```python
from build123d import *

# Parameters (mm, degrees)
SKETCH_1_R          = 7
EXTRUDE_1_DEPTH     = 3
SKETCH_2_R          = 6
EXTRUDE_2_DEPTH     = 8
SKETCH_3_R          = 7
EXTRUDE_3_DEPTH     = 3
CHAMFER_1_SIZE      = 2.144506921
CHAMFER_1_SIZE_2    = 1
CHAMFER_2_SIZE      = 2.144506921
CHAMFER_2_SIZE_2    = 1
SKETCH_4_R          = 5.9
EXTRUDE_4_DEPTH     = 2.2
EXTRUDE_START       = 2.2
SKETCH_5_R          = 5.9
EXTRUDE_5_DEPTH     = 2.2
SKETCH_6_W          = 6.5
SKETCH_6_H          = 6.5
CUT_EXTRUDE_1_DEPTH = 4
SKETCH_7_W          = 6.5
SKETCH_7_H          = 6.5
CUT_EXTRUDE_2_DEPTH = 4
SKETCH_8_R          = 1.2
CUT_EXTRUDE_3_DEPTH = 18.474552927


with BuildPart() as part:
    # Эскиз1 → Бобышка-Вытянуть1 (new body)
    with BuildSketch(Plane(origin=(0, 0, 0), x_dir=(1, 0, 0), z_dir=(0, 1, 0))):
        with Locations(Location((0, 0, 0), (0, 0, 270))):
            Circle(SKETCH_1_R)
    extrude(amount=EXTRUDE_1_DEPTH)

    # Эскиз2 → Бобышка-Вытянуть2 (add)
    with BuildSketch(Plane(origin=(0, 3, 0), x_dir=(1, 0, 0), z_dir=(0, 1, 0))):
        with Locations(Location((0, 0, 0), (0, 0, 270))):
            Circle(SKETCH_2_R)
    extrude(amount=EXTRUDE_2_DEPTH)

    # Эскиз3 → Бобышка-Вытянуть3 (add)
    with BuildSketch(Plane(origin=(0, 11, 0), x_dir=(1, 0, 0), z_dir=(0, 1, 0))):
        with Locations(Location((0, 0, 0), (0, 0, 270))):
            Circle(SKETCH_3_R)
    extrude(amount=EXTRUDE_3_DEPTH)

    # Фаска1
    # the kernel refuses this chamfer: 2.144506921, 1 mm, written as the material it adds along each edge
    with BuildSketch(Plane(origin=(0, 3, 0), x_dir=(0, 0, 1), z_dir=(-1, 0, 0))) as chamfer_1_piece_1_section:
        Polygon((6, CHAMFER_1_SIZE), (6 + CHAMFER_1_SIZE_2, 0), (6, 0), align=None)
    chamfer_1_piece_1 = revolve(axis=Axis((0, 3, 0), (0, 1, 0)), mode=Mode.PRIVATE)
    chamfer_1_piece_1 = chamfer_1_piece_1 & Plane(origin=(0, 4.095664656, 0), x_dir=(0, 0, 1), z_dir=(0, -1, 0)) * Cylinder(7, 28, mode=Mode.PRIVATE)
    add(chamfer_1_piece_1)

    # Фаска2
    # the kernel refuses this chamfer: 2.144506921, 1 mm, written as the material it adds along each edge
    with BuildSketch(Plane(origin=(0, 11, 0), x_dir=(0, 0, 1), z_dir=(-1, 0, 0))) as chamfer_2_piece_1_section:
        Polygon((6, -CHAMFER_2_SIZE), (6 + CHAMFER_2_SIZE_2, 0), (6, 0), align=None)
    chamfer_2_piece_1 = revolve(axis=Axis((0, 11, 0), (0, 1, 0)), mode=Mode.PRIVATE)
    chamfer_2_piece_1 = chamfer_2_piece_1 & Plane(origin=(0, 9.904335344, 0), x_dir=(0, 0, 1), z_dir=(0, -1, 0)) * Cylinder(7, 28, mode=Mode.PRIVATE)
    add(chamfer_2_piece_1)

    # Эскиз4 → Бобышка-Вытянуть4 (add)
    with BuildSketch(Plane(origin=(0, 14, 0), x_dir=(1, 0, 0), z_dir=(0, 1, 0))):
        with Locations(Location((0, 0, 0), (0, 0, 270))):
            Circle(SKETCH_4_R)
    extrude(amount=EXTRUDE_4_DEPTH)

    # Эскиз5 → Бобышка-Вытянуть5 (add)
    with BuildSketch(Plane.XZ.offset(EXTRUDE_START)):
        with Locations(Location((0, 0, 0), (0, 0, 90))):
            Circle(SKETCH_5_R)
    extrude(amount=-EXTRUDE_5_DEPTH)

    # Эскиз6 → Вырез-Вытянуть1 (cut)
    with BuildSketch(Plane(origin=(0, 16.2, 0), x_dir=(1, 0, 0), z_dir=(0, 1, 0))):
        Rectangle(SKETCH_6_W, SKETCH_6_H)
    extrude(amount=-CUT_EXTRUDE_1_DEPTH, mode=Mode.SUBTRACT)

    # Эскиз7 → Вырез-Вытянуть2 (cut)
    with BuildSketch(Plane.XZ.offset(2.2)):
        Rectangle(SKETCH_7_W, SKETCH_7_H)
    extrude(amount=-CUT_EXTRUDE_2_DEPTH, mode=Mode.SUBTRACT)

    # Эскиз8 → Вырез-Вытянуть3 (cut, through all)
    with BuildSketch(Plane.XZ.offset(-1.8)):
        with Locations(Location((0, 0, 0), (0, 0, 270))):
            Circle(SKETCH_8_R)
    extrude(amount=-CUT_EXTRUDE_3_DEPTH, mode=Mode.SUBTRACT)


solid = part.part
```
Verification items for the finished model (mm, model axes). A direction names the side the tool comes from. Coordinates: 2 decimals unless noted, no trailing zeros. Write each loop counter-clockwise with the first axis right and the second up, starting at its lowest first coordinate (ties: lowest second). Pieces come first, ordered by that corner, then holes. Notation, with made-up numbers: M 17,-11 L 67,-11 A23 cw 67,2 Z; hole C 76.25,30 d10. An arc over 180 degrees is marked long. One line per item, written item: value.
Item 1: Scan lines: line 1 along X through (y, z) = (7.5, 0); line 2 along Y through (x, z) = (-1.25, -2); line 3 along X through (y, z) = (15.5, -1.5). Record each from-to range of solid material in increasing order.
Check sheet entries:
line 1: x = -6 to -1.2, 1.2 to 6
line 2: y = 1.8 to 12.2
line 3: x = -5.71 to -3.25, 3.25 to 5.71
Item 2: Access from +Z, -Z, +X, -X, +Y, -Y to the whole of each face (thin tool, end or side, straight path). Record for faces 1 (the flat face through (3.25, 14, 0)), 2 (the flat face through (0, 0, 3.25)), 3 (the cylindrical face through (1.802, 6.974, 5.723)).
Check sheet entries:
face 1: +Y
face 2: -Y
face 3: none
Item 3: Gauge pin test, flat ends, axial feed: pin 1 Ø1.2 at (y, z) = (15, -0.5) entering from -X; pin 2 Ø8 at (x, y) = (3, 11.5) entering from -Z; pin 3 Ø4 at (y, z) = (10.5, -4) entering from +X; pin 4 Ø4 at (x, z) = (0, 0.5) entering from -Y. Record the tip position at first contact, or that the pin passes through.
Check sheet entries:
pin 1: stops at x = -5.9
pin 2: stops at z = -7
pin 3: stops at x = 6.69
pin 4: stops at y = 1.8
Item 4: Section check C-C, the plane y = 13. Record the boundary of the cut face in (x, z), plus the area to 3 significant figures.
Check sheet entries:
outline: C 0,0 d14; hole M -3.25,-3.25 L 3.25,-3.25 L 3.25,3.25 L -3.25,3.25 Z
area: 112 mm^2
Item 5: Mould release check, pull along Z, two halves, no side actions. Record for faces 4 (the flat face through (4, -2.2, 0)), 5 (the cylindrical face through (-5.76, 15.08, -1.28)), 6 (the flat face through (3.25, 0, 0)): pulls with the +Z half, pulls with the -Z half, needs draft (parallel to the pull), parting line crosses it, or undercut.
Check sheet entries:
face 4: needs draft
face 5: parting line crosses it
face 6: undercut
Item 6: Section check D-D, the plane y = 10.75. Record the boundary of the cut face in (x, z).
Check sheet entries:
outline: C 0,0 d13.77; hole C 0,0 d2.4
